Verification items for the finished model (mm, model axes). Face numbers are marked on the shaded views. Round coordinates to 2 decimals unless told otherwise and drop trailing zeros. Write each loop counter-clockwise with the first axis right and the second up, starting at its lowest first coordinate (ties: lowest second). Pieces come first, ordered by that corner, then holes. Notation, with made-up numbers: M 64,26.5 L 96,26.5 A13 cw 96,42.5 Z; hole C 61,-22 d1. An arc over 180 degrees is marked long. One line per item, written item: value. Start each with the question number.
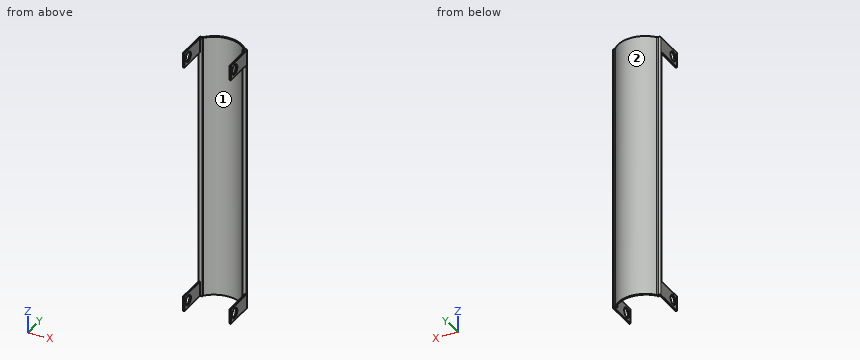
from build123d import *

# Parameters (mm, degrees)
AUFSATZ_LINEAR_AUSTRAGEN1_DEPTH = 180
DURCHGANGSLOCH_F_R_M61_D        = 6.6
SKIZZE4_W                       = 160
SKIZZE4_H                       = 20
SCHNITT_LINEAR_AUSTRAGEN1_DEPTH = 185.137137843
VERRUNDUNG1_R                   = 1


with BuildPart() as part:
    # Skizze1 → Aufsatz-Linear austragen1 (new body)
    with BuildSketch(Plane.XY):
        with BuildLine():
            Line((-16.15, 0), (-14.230984974, 0))
            ThreePointArc((-14.230984974, 0), (0, 6.679295001), (14.230984974, 0))
            Line((14.230984974, 0), (16.15, 0))
            Line((16.15, 0), (16.15, -21.521977909))
            Line((16.15, -21.521977909), (15.15, -21.521977909))
            Line((15.15, -21.521977909), (15.15, -1.521977909))
            Line((15.15, -1.521977909), (15, -1.521977909))
            Line((15, -1.521977909), (13.59375, -1.521977909))
            Line((13.59375, -1.521977909), (13.59375, -0.521977909))
            ThreePointArc((13.59375, -0.521977909), (0, 5.679295001), (-13.59375, -0.521977909))
            Line((-13.59375, -0.521977909), (-13.59375, -1.521977909))
            Line((-13.59375, -1.521977909), (-15, -1.521977909))
            Line((-15, -1.521977909), (-15.15, -1.521977909))
            Line((-15.15, -1.521977909), (-15.15, -21.521977909))
            Line((-15.15, -21.521977909), (-16.15, -21.521977909))
            Line((-16.15, -21.521977909), (-16.15, 0))
        make_face()
    extrude(amount=AUFSATZ_LINEAR_AUSTRAGEN1_DEPTH)

    # Durchgangsloch für M61 (through all)
    with Locations(Plane(origin=(-16.15, 0, 0), x_dir=(0, 0, -1), z_dir=(-1, 0, 0))):
        with Locations((-5, 16.521977909)):
            durchgangsloch_f_r_m61 = Hole(DURCHGANGSLOCH_F_R_M61_D / 2)

    # Spiegeln1: Durchgangsloch für M61 across plane
    add(durchgangsloch_f_r_m61.mirror(Plane.XY.offset(90)), mode=Mode.SUBTRACT)

    # Skizze4 → Schnitt-Linear austragen1 (cut, through all)
    with BuildSketch(Plane(origin=(16.15, 0, 0), x_dir=(0, 0, -1), z_dir=(1, 0, 0))):
        with Locations((-90, -11.521977909)):
            Rectangle(SKIZZE4_W, SKIZZE4_H)
    extrude(amount=-SCHNITT_LINEAR_AUSTRAGEN1_DEPTH, mode=Mode.SUBTRACT)

    # Verrundung1
    verrundung1_edges = [part.edges().sort_by_distance(p)[0] for p in [
        (14.230984974, 0, 90),
        (16.15, 0, 90),
        (-16.15, 0, 90),
        (-14.230984974, 0, 90),
    ]]
    fillet(verrundung1_edges, radius=VERRUNDUNG1_R)


solid = part.part
1) Cross-section at A-A (y = -9.5). Record the boundary of the cut face in (x, z), then the cut area to 3 significant figures.
2) Cross-section at B-B (z = 5). Record the boundary of the cut face in (x, y), then the cut area to 3 significant figures.
3) Cross-section at C-C (z = 97.5). Record the boundary of the cut face in (x, y).
4) Mould release check, pull along X, two halves, no side actions. Record for the marked faces 1 and 2: pulls with the +X half, pulls with the -X half, needs draft (parallel to the pull), parting line crosses it, or undercut.
5) Thickness scan on line 1 (Y direction, x = -15.65, z = 175); line 2 (X direction, y = 1, z = 154.5); line 3 (X direction, y = 2.25, z = 36.5). Record the ranges inside material, lowest first.
6) Cross-section at D-D (x = 0). Record the boundary of the cut face in (y, z).
7) Gauge pin test, flat ends, axial feed: pin 1 Ø5 at (x, y) = (8, -1.5) entering from +Z; pin 2 Ø1 at (x, z) = (0, 138.5) entering from -Y; pin 3 Ø1.5 at (y, z) = (3, 67) entering from +X; pin 4 Ø2 at (x, z) = (-15.5, 73) entering from -Y. Record the tip position at first contact, or that the pin passes through.
Results below:
1. outline: M -16.15,0 L -15.15,0 L -15.15,10 L -16.15,10 Z; M -16.15,170 L -15.15,170 L -15.15,180 L -16.15,180 Z; M 15.15,0 L 16.15,0 L 16.15,10 L 15.15,10 Z; M 15.15,170 L 16.15,170 L 16.15,180 L 15.15,180 Z
1. area: 40.0 mm²
2. outline: M -16.15,-21.52 L -15.15,-21.52 L -15.15,-19.82 L -16.15,-19.82 Z; M -16.15,-13.22 L -15.15,-13.22 L -15.15,-1.52 L -13.59,-1.52 L -13.59,-0.52 A18 cw 13.59,-0.52 L 13.59,-1.52 L 15.15,-1.52 L 15.15,-13.22 L 16.15,-13.22 L 16.15,-1 A1 ccw 15.15,0 L 14.69,0 A1 cw 13.94,0.34 A18.5 ccw -13.94,0.34 A1 cw -14.69,0 L -15.15,0 A1 ccw -16.15,-1 Z; M 15.15,-21.52 L 16.15,-21.52 L 16.15,-19.82 L 15.15,-19.82 Z
2. area: 63.6 mm²
3. outline: M -16.15,-1.52 L -13.59,-1.52 L -13.59,-0.52 A18 cw 13.59,-0.52 L 13.59,-1.52 L 16.15,-1.52 L 16.15,-1 A1 ccw 15.15,0 L 14.69,0 A1 cw 13.94,0.34 A18.5 ccw -13.94,0.34 A1 cw -14.69,0 L -15.15,0 A1 ccw -16.15,-1 Z
4. face 1: undercut
4. face 2: parting line crosses it
5. line 1: y = -21.52 to -19.82, -13.22 to -0.13
5. line 2: x = -13.34 to -12.11, 12.11 to 13.34
5. line 3: x = -12.01 to -10.57, 10.57 to 12.01
6. outline: M 5.68,0 L 6.68,0 L 6.68,180 L 5.68,180 Z
7. pin 1: passes through
7. pin 2: stops at y = 5.67
7. pin 3: stops at x = 12.01
7. pin 4: stops at y = -1.52
